```python
from build123d import *

# Parameters (mm, degrees)
SKETCH2_W           = 58.42
SKETCH2_H           = 25.4
BOSS_EXTRUDE1_DEPTH = 36.7
CUT_EXTRUDE1_REACH  = 75.518
SKETCH3_W           = 4.252
SKETCH3_H           = 23.4
SKETCH3_W_2         = 28.448
SKETCH4_W           = 8.16
SKETCH4_H           = 23.4
CUT_EXTRUDE3_DEPTH  = 2
FILLET1_R           = 1
CUT_EXTRUDE5_REACH  = 73.491
SKETCH5_W           = 40.82
SKETCH5_H           = 23.4
SKETCH6_W           = 2.06
SKETCH6_H           = 2.548
CUT_EXTRUDE6_DEPTH  = 2
CUT_EXTRUDE7_DEPTH  = 2
FILLET2_R           = 1
SKETCH8_R           = 1.5
CUT_EXTRUDE8_DEPTH  = 2
SKETCH9_R           = 2.25
SKETCH9_R_2         = 4
SKETCH9_R_3         = 1.5
CUT_EXTRUDE9_DEPTH  = 2
SKETCH10_R          = 2.25
CUT_EXTRUDE10_DEPTH = 2
FILLET3_R           = 1


with BuildPart() as part:
    # Sketch2 → Boss-Extrude1 (new body)
    with BuildSketch(Plane.XY):
        with Locations((29.21, 12.7)):
            Rectangle(SKETCH2_W, SKETCH2_H)
    extrude(amount=BOSS_EXTRUDE1_DEPTH)

    # Sketch3 → Cut-Extrude1 (cut, up to next)
    with BuildSketch(Plane(origin=(58.42, 0, 0), x_dir=(0, 0, -1), z_dir=(1, 0, 0)), mode=Mode.PRIVATE) as cut_extrude1_sk1:
        with Locations((-2.126, 13.7)):
            Rectangle(SKETCH3_W, SKETCH3_H)
    cut_extrude1_tool1 = extrude(cut_extrude1_sk1.sketch, amount=-CUT_EXTRUDE1_REACH, mode=Mode.PRIVATE) & part.part
    # Sketch3 → Cut-Extrude1 (cut, up to next)
    with BuildSketch(Plane(origin=(58.42, 0, 0), x_dir=(0, 0, -1), z_dir=(1, 0, 0)), mode=Mode.PRIVATE) as cut_extrude1_sk2:
        with Locations((-20.476, 13.7)):
            Rectangle(SKETCH3_W_2, SKETCH3_H)
    cut_extrude1_tool2 = extrude(cut_extrude1_sk2.sketch, amount=-CUT_EXTRUDE1_REACH, mode=Mode.PRIVATE) & part.part
    add(cut_extrude1_tool1.solids().sort_by_distance((58.42, 13.7, 2.126))[0], mode=Mode.SUBTRACT)
    add(cut_extrude1_tool2.solids().sort_by_distance((58.42, 13.7, 20.476))[0], mode=Mode.SUBTRACT)

    # Sketch4 → Cut-Extrude3 (cut)
    with BuildSketch(Plane.XY.offset(36.7)):
        with Locations((4.08, 13.7)):
            Rectangle(SKETCH4_W, SKETCH4_H)
        with Locations((54.34, 13.7)):
            Rectangle(SKETCH4_W, SKETCH4_H)
    extrude(amount=-CUT_EXTRUDE3_DEPTH, mode=Mode.SUBTRACT)

    # Fillet1
    fillet1_edges = [part.edges().sort_by_distance(p)[0] for p in [
        (29.21, 2, 34.7),
        (8.16, 25.4, 35.7),
        (50.26, 25.4, 35.7),
        (29.21, 0, 36.7),
    ]]
    fillet(fillet1_edges, radius=FILLET1_R)

    # Sketch5 → Cut-Extrude5 (cut, up to next)
    with BuildSketch(Plane(origin=(0, 0, 4.252), x_dir=(-1, 0, 0), z_dir=(0, 0, -1)), mode=Mode.PRIVATE) as cut_extrude5_sk1:
        with Locations((-29.21, 13.7)):
            Rectangle(SKETCH5_W, SKETCH5_H)
    cut_extrude5_tool1 = extrude(cut_extrude5_sk1.sketch, amount=-CUT_EXTRUDE5_REACH, mode=Mode.PRIVATE) & part.part
    add(cut_extrude5_tool1.solids().sort_by_distance((29.21, 13.7, 4.252))[0], mode=Mode.SUBTRACT)

    # Sketch6 → Cut-Extrude6 (cut)
    with BuildSketch(Plane(origin=(0, 2, 0), x_dir=(1, 0, 0), z_dir=(0, 1, 0))):
        Polygon((10.86, -6.252), (10.86, 0), (0, 0), (0, -4.252), (8.8, -4.252), (8.8, -6.252), align=None)
        Polygon((58.42, 0), (47.56, 0), (47.56, -6.252), (49.62, -6.252), (49.62, -4.252), (58.42, -4.252), align=None)
        with Locations((48.59, -7.526)):
            Rectangle(SKETCH6_W, SKETCH6_H)
        with Locations((9.83, -7.526)):
            Rectangle(SKETCH6_W, SKETCH6_H)
    extrude(amount=-CUT_EXTRUDE6_DEPTH, mode=Mode.SUBTRACT)

    # Sketch7 → Cut-Extrude7 (cut)
    with BuildSketch(Plane(origin=(0, 2, 0), x_dir=(1, 0, 0), z_dir=(0, 1, 0))):
        Polygon((0, -36.7), (8.16, -36.7), (8.16, -33.7), (8.16, -28.552), (0, -28.552), align=None)
        Polygon((58.42, -36.7), (58.42, -28.552), (50.26, -28.552), (50.26, -33.7), (50.26, -36.7), align=None)
    extrude(amount=-CUT_EXTRUDE7_DEPTH, mode=Mode.SUBTRACT)

    # Fillet2
    fillet2_edges = [part.edges().sort_by_distance(p)[0] for p in [
        (49.62, 25.4, 5.252),
        (8.8, 25.4, 5.252),
        (47.56, 1, 0),
        (10.86, 1, 0),
        (0, 1, 28.552),
        (58.42, 1, 28.552),
        (58.42, 25.4, 5.252),
        (0, 25.4, 5.252),
    ]]
    fillet(fillet2_edges, radius=FILLET2_R)

    # Sketch8 → Cut-Extrude8 (cut)
    with BuildSketch(Plane.XY.offset(36.7)):
        with Locations((19.091571086, 13.4)):
            Circle(SKETCH8_R)
        with Locations((19.091571086, 20.9)):
            Circle(SKETCH8_R)
        with Locations((26.591571086, 13.4)):
            Circle(SKETCH8_R)
        with Locations((19.091571086, 5.9)):
            Circle(SKETCH8_R)
        with Locations((11.591571086, 13.4)):
            Circle(SKETCH8_R)
        with Locations((39.091571086, 13.4)):
            Circle(SKETCH8_R)
        with Locations((39.091571086, 5.9)):
            Circle(SKETCH8_R)
        with Locations((31.591571086, 13.4)):
            Circle(SKETCH8_R)
        with Locations((39.091571086, 20.9)):
            Circle(SKETCH8_R)
        with Locations((46.591571086, 13.4)):
            Circle(SKETCH8_R)
    extrude(amount=-CUT_EXTRUDE8_DEPTH, mode=Mode.SUBTRACT)

    # Sketch9 → Cut-Extrude9 (cut)
    with BuildSketch(Plane(origin=(0, 2, 0), x_dir=(1, 0, 0), z_dir=(0, 1, 0))):
        with Locations(Location((4.21, -14.552, 0), (0, 0, 270))):
            Circle(SKETCH9_R)
        with Locations(Location((4.21, -24.552, 0), (0, 0, 270))):
            Circle(SKETCH9_R)
        with Locations(Location((54.21, -14.552, 0), (0, 0, 270))):
            Circle(SKETCH9_R)
        with Locations(Location((54.21, -24.552, 0), (0, 0, 270))):
            Circle(SKETCH9_R)
        with Locations(Location((29.21, -24.552, 0), (0, 0, 270))):
            Circle(SKETCH9_R_2)
        with Locations(Location((29.21, -17.052, 0), (0, 0, 270))):
            Circle(SKETCH9_R_3)
        with Locations(Location((36.71, -24.552, 0), (0, 0, 270))):
            Circle(SKETCH9_R_3)
        with Locations(Location((29.21, -32.052, 0), (0, 0, 270))):
            Circle(SKETCH9_R_3)
        with Locations(Location((21.71, -24.552, 0), (0, 0, 270))):
            Circle(SKETCH9_R_3)
        with Locations(Location((39.21, -14.552, 0), (0, 0, 270))):
            Circle(SKETCH9_R_2)
        with Locations(Location((19.21, -14.552, 0), (0, 0, 270))):
            Circle(SKETCH9_R_2)
        with Locations(Location((31.71, -14.552, 0), (0, 0, 270))):
            Circle(SKETCH9_R_3)
        with Locations(Location((39.21, -7.052, 0), (0, 0, 270))):
            Circle(SKETCH9_R_3)
        with Locations(Location((46.71, -14.552, 0), (0, 0, 270))):
            Circle(SKETCH9_R_3)
        with Locations(Location((39.21, -22.052, 0), (0, 0, 270))):
            Circle(SKETCH9_R_3)
        with Locations(Location((26.71, -14.552, 0), (0, 0, 270))):
            Circle(SKETCH9_R_3)
        with Locations(Location((19.21, -22.052, 0), (0, 0, 270))):
            Circle(SKETCH9_R_3)
        with Locations(Location((11.71, -14.552, 0), (0, 0, 270))):
            Circle(SKETCH9_R_3)
        with Locations(Location((19.21, -7.052, 0), (0, 0, 270))):
            Circle(SKETCH9_R_3)
    extrude(amount=-CUT_EXTRUDE9_DEPTH, mode=Mode.SUBTRACT)

    # Sketch10 → Cut-Extrude10 (cut)
    with BuildSketch(Plane(origin=(0, 0, 4.252), x_dir=(-1, 0, 0), z_dir=(0, 0, -1))):
        with Locations(Location((-4.21, 18.11, 0), (0, 0, 90))):
            Circle(SKETCH10_R)
        with Locations(Location((-54.21, 18.11, 0), (0, 0, 90))):
            Circle(SKETCH10_R)
        with Locations(Location((-54.21, 8.11, 0), (0, 0, 90))):
            Circle(SKETCH10_R)
        with Locations(Location((-4.21, 8.11, 0), (0, 0, 90))):
            Circle(SKETCH10_R)
    extrude(amount=-CUT_EXTRUDE10_DEPTH, mode=Mode.SUBTRACT)

    # Fillet3
    fillet3_edges = [part.edges().sort_by_distance(p)[0] for p in [
        (54.02, 2, 6.252),
        (4.4, 2, 6.252),
    ]]
    fillet(fillet3_edges, radius=FILLET3_R)


solid = part.part
```
For this review, take the finished solid that the model builds, in its own axes (mm). A direction names the side the tool comes from. Coordinates: 2 decimals unless noted, no trailing zeros. Order: outer loops, then holes, each group sorted by start corner. A loop starts at its lowest first (then second) coordinate and runs counter-clockwise, first axis right, second up. Notation, with made-up numbers: (7, 15.25) -> (26, 15.25) arc R28 cw to (26, 50.25) -> close; hole circle Ø5 at (-15.5, 63). An arc over 180 degrees is marked (long way). Answer as CSV lines item,"result".
Q1. For faces 1 (the face through (10, 1, 8.8)), 2 (the face through (35.246, 1.014, 24.227)), 3 (the face through (4, 13, 4.252)), list the 3-axis set-ups (+Z, -Z, +X, -X, +Y, -Y) from which the entire face can be reached by the end or side of a thin tool; tool diameter is ignored.
Model answer:
face 1,"-Z, +Y, -Y"
face 2,"+Y, -Y"
face 3,"-Z, -X, +Y, -Y"
Q2. Draft analysis for pull direction X (two halves, no side actions). For faces 4 (the face through (29, 25.4, 36)), 5 (the face through (8.16, 10, 35)), 6 (the face through (45.093, 13.466, 35.714)), 7 (the face through (37.9, 12.49, 35.71)), state which applies: released by +X, released by -X, zero draft, split by the parting line, or undercut.
Model answer:
face 4,"zero draft"
face 5,"released by -X"
face 6,"undercut"
face 7,"undercut"
Q3. Wall thickness on line 1 along Y through (x, z) = (55, 19); line 2 along Z through (x, y) = (50, 13); line 3 along Z through (x, y) = (9, 12.75): over which ranges is each line inside the solid? List them lowest first. Write a range as [from, to].
Model answer:
line 1,"y = [0, 2]"
line 2,"z = [4.25, 6.25], [34.7, 36.7]"
line 3,"z = [34.7, 36.7]"
Q4. We need section A-A (y = 8.11). State the section outline as (x, z) points.
Model answer:
outline,"(0, 4.25) -> (1.96, 4.25) -> (1.96, 6.25) -> (0, 6.25) -> close; (6.46, 4.25) -> (8.8, 4.25) -> (8.8, 6.25) -> (6.46, 6.25) -> close; (8.16, 34.7) -> (50.26, 34.7) -> (50.26, 36.7) -> (8.16, 36.7) -> close; (49.62, 4.25) -> (51.96, 4.25) -> (51.96, 6.25) -> (49.62, 6.25) -> close; (56.46, 4.25) -> (58.42, 4.25) -> (58.42, 6.25) -> (56.46, 6.25) -> close"
Q5. We need section B-B (x = 4.21). State the section outline as (y, z) points, plus the area to 3 significant figures.
Model answer:
outline,"(0, 4.25) -> (5.86, 4.25) -> (5.86, 6.25) -> (3, 6.25) arc R1 cw to (2, 7.25) -> (2, 12.3) -> (0, 12.3) -> close; (0, 16.8) -> (2, 16.8) -> (2, 22.3) -> (0, 22.3) -> close; (0, 26.8) -> (2, 26.8) -> (2, 28.55) -> (0, 28.55) -> close; (10.36, 4.25) -> (15.86, 4.25) -> (15.86, 6.25) -> (10.36, 6.25) -> close; (20.36, 4.25) -> (25.4, 4.25) -> (25.4, 6.25) -> (20.36, 6.25) -> close"
area,"59.6 mm2"
Q6. Clearance check with flat-ended pins moving along their axes: pin 1 Ø1.8 at (x, y) = (19.09, 13.4) entering from -Z; pin 2 Ø0.6 at (x, y) = (53.5, 1) entering from +Z; pin 3 Ø5 at (x, z) = (4.21, 14.552) entering from +Y; pin 4 Ø1 at (x, y) = (10, 1) entering from -Z. State where each tip first meets the part, or that it passes through.
Model answer:
pin 1,"passes through"
pin 2,"stops at z = 28.55"
pin 3,"stops at y = 2"
pin 4,"stops at z = 8.8"
Q7. We need section D-D (x = 36.71). State the section outline as (y, z) points.
Model answer:
outline,"(0, 0) -> (2, 0) -> (2, 11.43) -> (0, 11.43) -> close; (0, 17.67) -> (2, 17.67) -> (2, 23.05) -> (0, 23.05) -> close; (0, 26.05) -> (2, 26.05) -> (2, 33.7) arc R1 cw to (3, 34.7) -> (25.4, 34.7) -> (25.4, 36.7) -> (1, 36.7) arc R1 ccw to (0, 35.7) -> close"
Q8. We need section C-C (y = 23.25). State the section outline as (x, z) points, plus the area to 3 significant figures.
Model answer:
outline,"(0, 4.25) -> (8.8, 4.25) -> (8.8, 6.25) -> (0, 6.25) -> close; (8.16, 34.7) -> (50.26, 34.7) -> (50.26, 36.7) -> (8.16, 36.7) -> close; (49.62, 4.25) -> (58.42, 4.25) -> (58.42, 6.25) -> (49.62, 6.25) -> close"
area,"119 mm2"
